Part model, mm, in its own coordinate system. Face numbers are marked on the shaded views. A direction names the side the tool comes from. Coordinates: 2 decimals unless noted, no trailing zeros. Order: outer loops, then holes, each group sorted by start corner. A loop starts at its lowest first (then second) coordinate and runs counter-clockwise, first axis right, second up.
1) Tool access for the marked faces 4, 5 and 6: list every direction of +Z, -Z, +X, -X, +Y, -Y with a clear straight run to the whole face (end or side of a thin tool).
2) Mould opens along Y. For the marked faces 1, 2 and 3 say: +Y half, -Y half, draft (parallel to the pull), parting line (faces both ways), or undercut.
3) Pin check, flat tips, straight feed: pin 1 Ø4.5 at (x, z) = (-22.5, -0.5) entering from +Y; pin 2 Ø1 at (y, z) = (6, -7) entering from +X; pin 3 Ø3 at (y, z) = (33, -4) entering from +X. Stop position of each tip, or through.
4) Cut at A-A (y = -13.5). List the corners of the cut face in (x, z).
5) Cut at D-D (z = -7). List the corners of the cut face in (x, y) (1 decimal).
6) Wall check: L1, parallel to X at y = -24.5, z = -2; L2, parallel to Z at x = 0, y = 22; L3, parallel to X at y = -2, z = 0.5. Give the ranges that are in metal, low to high.
7) Cut at B-B (x = 0). List the corners of the cut face in (y, z).
8) Cut at C-C (z = 0). List the corners of the cut face in (x, y) (1 decimal), and give its area (3 significant figures).
```python
from build123d import *

# Parameters (mm, degrees)
BOSS_EXTRUDE1_DEPTH = 9
FILLET1_R           = 4
FILLET2_R           = 2
HOLE1_D             = 12


with BuildPart() as part:
    # Sketch1 → Boss-Extrude1 (new, symmetric)
    with BuildSketch(Plane.XY):
        with BuildLine():
            Line((-18, 0), (-24, 0))
            Line((-24, 0), (-24, -19))
            Line((-24, -19), (-20, -19))
            Line((-20, -19), (-20, -30))
            Line((-20, -30), (-33, -30))
            Line((-33, -30), (-33, 0))
            Line((-33, 0), (-30, 0))
            ThreePointArc((-30, 0), (-24.186773245, 17.748239349), (-9, 28.618176043))
            Line((-9, 28.618176043), (-9, 34))
            Line((-9, 34), (9, 34))
            Line((9, 34), (9, 28.618176043))
            ThreePointArc((9, 28.618176043), (24.186773245, 17.748239349), (30, 0))
            Line((30, 0), (33, 0))
            Line((33, 0), (33, -30))
            Line((33, -30), (20, -30))
            Line((20, -30), (20, -19))
            Line((20, -19), (24, -19))
            Line((24, -19), (24, 0))
            Line((24, 0), (18, 0))
            ThreePointArc((18, 0), (0, 18), (-18, 0))
        make_face()
    extrude(amount=BOSS_EXTRUDE1_DEPTH, both=True)

    # Fillet1
    fillet1_edges = [part.edges().sort_by_distance(p)[0] for p in [
        (-9, 28.618176043, 0),
        (9, 28.618176043, 0),
    ]]
    fillet(fillet1_edges, radius=FILLET1_R)

    # Fillet2
    fillet2_edges = [part.edges().sort_by_distance(p)[0] for p in [
        (30, 0, 0),
        (-30, 0, 0),
    ]]
    fillet(fillet2_edges, radius=FILLET2_R)

    # Hole1 (through all)
    with Locations(Plane(origin=(0, 34, 0), x_dir=(1, 0, 0), z_dir=(0, 1, 0))):
        with Locations((0, 0)):
            Hole(HOLE1_D / 2)


solid = part.part
```
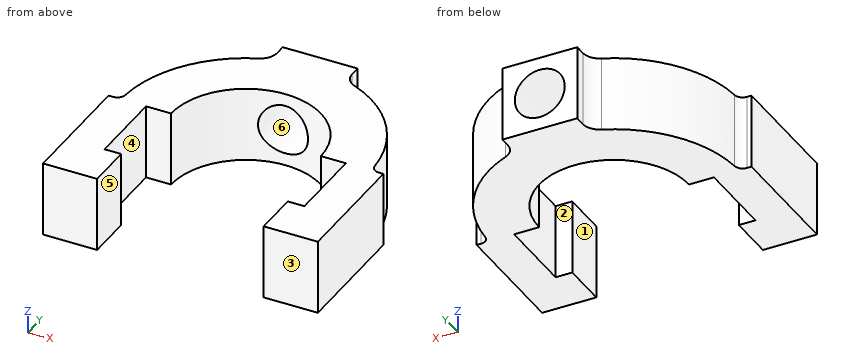
Geometry check:
1. face 4: +Z, -Z
1. face 5: +Z, -Z, -Y
1. face 6: +Y, -Y
2. face 1: draft
2. face 2: undercut
2. face 3: -Y half
3. pin 1: stops at y = 22.13
3. pin 2: stops at x = 29.49
3. pin 3: stops at x = 9
4. outline: (-33, -9) - (-24, -9) - (-24, 9) - (-33, 9) - close; (24, -9) - (33, -9) - (33, 9) - (24, 9) - close
5. outline: (-33, -30) - (-20, -30) - (-20, -19) - (-24, -19) - (-24, 0) - (-18, 0) arc R18 cw to (18, 0) - (24, 0) - (24, -19) - (20, -19) - (20, -30) - (33, -30) - (33, 0) - (31.9, 0) arc R2 cw to (29.9, 1.9) arc R30 ccw to (11.5, 27.7) arc R4 cw to (9, 31.4) - (9, 34) - (-9, 34) - (-9, 31.4) arc R4 cw to (-11.5, 27.7) arc R30 ccw to (-29.9, 1.9) arc R2 cw to (-31.9, 0) - (-33, 0) - close
6. L1: x = -33 to -20, 20 to 33
6. L2: z = -9 to -6, 6 to 9
6. L3: x = -33 to -24, 24 to 33
7. outline: (18, -9) - (34, -9) - (34, -6) - (18, -6) - close; (18, 6) - (34, 6) - (34, 9) - (18, 9) - close
8. outline: (-33, -30) - (-20, -30) - (-20, -19) - (-24, -19) - (-24, 0) - (-18, 0) arc R18 cw to (-6, 17) - (-6, 34) - (-9, 34) - (-9, 31.4) arc R4 cw to (-11.5, 27.7) arc R30 ccw to (-29.9, 1.9) arc R2 cw to (-31.9, 0) - (-33, 0) - close; (6, 17) arc R18 cw to (18, 0) - (24, 0) - (24, -19) - (20, -19) - (20, -30) - (33, -30) - (33, 0) - (31.9, 0) arc R2 cw to (29.9, 1.9) arc R30 ccw to (11.5, 27.7) arc R4 cw to (9, 31.4) - (9, 34) - (6, 34) - close
8. area: 1,420 mm2
